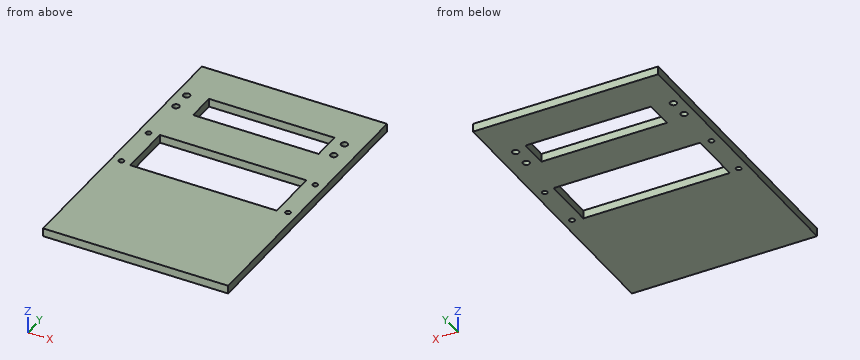
from build123d import *

# Parameters (mm, degrees)
SKETCH_W   = 90
SKETCH_H   = 140
SKETCH_R   = 1.25
SKETCH_R_2 = 1.6
SKETCH_W_2 = 71.2
SKETCH_H_2 = 26.2
SKETCH_W_3 = 61
SKETCH_H_3 = 14
PAD_DEPTH  = 4


with BuildPart() as part:
    # Sketch → Pad (new body)
    with BuildSketch(Plane.XY):
        Rectangle(SKETCH_W, SKETCH_H)
        with Locations((-40.5, 14.9)):
            Circle(SKETCH_R, mode=Mode.SUBTRACT)
        with Locations((-40.5, -9.1)):
            Circle(SKETCH_R, mode=Mode.SUBTRACT)
        with Locations((40.5, 14.9)):
            Circle(SKETCH_R, mode=Mode.SUBTRACT)
        with Locations((40.5, -9.1)):
            Circle(SKETCH_R, mode=Mode.SUBTRACT)
        with Locations((-40.1, 47.7)):
            Circle(SKETCH_R_2, mode=Mode.SUBTRACT)
        with Locations((-40.1, 38.3)):
            Circle(SKETCH_R_2, mode=Mode.SUBTRACT)
        with Locations((36.6, 47.7)):
            Circle(SKETCH_R_2, mode=Mode.SUBTRACT)
        with Locations((36.6, 38.3)):
            Circle(SKETCH_R_2, mode=Mode.SUBTRACT)
        with Locations((0, 2.9)):
            Rectangle(SKETCH_W_2, SKETCH_H_2, mode=Mode.SUBTRACT)
        with Locations((0, 43)):
            Rectangle(SKETCH_W_3, SKETCH_H_3, mode=Mode.SUBTRACT)
    extrude(amount=PAD_DEPTH)


solid = part.part
CAD build for the part. Positions are in the model's coordinates, mm. Give positions to 0.01 mm unless a question says otherwise; leave off trailing zeros. Loops run counter-clockwise (first coordinate to the right, second up) from the corner with the lowest first, then second, coordinate; pieces in that order, holes last. Notation, with made-up numbers: M -17.5,78.5 L 25.5,78.5 A16 cw 25.5,84.5 Z; hole C -0.5,52 d4. An arc over 180 degrees is marked long. Answer in a Markdown table with one row per item. Add a question column.
Item 1: Band-saw the part on D-D on y = 4.5. Give the cut face in (x, z).
Item 2: Band-saw the part on A-A on z = 0.9. Give the number of separate pieces and of enclosed holes in the cut face, then the cut area to 3 significant figures.
Item 3: Band-saw the part on C-C on x = -12. Give the cut face in (y, z).
Item 4: Probe probe 1 along Y at (x, z) = (-7, 1.7); probe 2 along Y at (x, z) = (-40.1, 1.55); probe 3 along X at (y, z) = (45.5, 2.1). List the from-to ranges inside material, lowest first.
Item 5: Band-saw the part on B-B on y = 38.3. Give the cut face in (x, z), then the cut area to 3 significant figures.
Reply:
| question | item | result |
|---|---|---|
| 1 | outline | M -45,0 L -35.6,0 L -35.6,4 L -45,4 Z; M 35.6,0 L 45,0 L 45,4 L 35.6,4 Z |
| 2 | separate pieces | 1 |
| 2 | enclosed holes | 10 |
| 2 | area | 9,830 mm^2 |
| 3 | outline | M -70,0 L -10.2,0 L -10.2,4 L -70,4 Z; M 16,0 L 36,0 L 36,4 L 16,4 Z; M 50,0 L 70,0 L 70,4 L 50,4 Z |
| 4 | probe 1 | y = -70 to -10.2, 16 to 36, 50 to 70 |
| 4 | probe 2 | y = -70 to -10.28, -7.92 to 13.72, 16.08 to 36.7, 39.9 to 46.1, 49.3 to 70 |
| 4 | probe 3 | x = -45 to -30.5, 30.5 to 45 |
| 5 | outline | M -45,0 L -41.7,0 L -41.7,4 L -45,4 Z; M -38.5,0 L -30.5,0 L -30.5,4 L -38.5,4 Z; M 30.5,0 L 35,0 L 35,4 L 30.5,4 Z; M 38.2,0 L 45,0 L 45,4 L 38.2,4 Z |
| 5 | area | 90.4 mm^2 |
